The drawing under review shows one solid part. Ordinate dimensions are in mm from its lowest x, y, z. Round coordinates to 2 decimals unless told otherwise and drop trailing zeros. Write each loop counter-clockwise with the first axis right and the second up, starting at its lowest first coordinate (ties: lowest second). Pieces come first, ordered by that corner, then holes.
Item 1: Add section A-A (y = 9). State how many separate pieces and enclosed holes the cut face has, plus the area to 3 significant figures.
Item 2: Add section D-D (z = 6.55). Give the boundary of the cut face in (x, y), plus the area to 3 significant figures.
Item 3: Add section C-C (y = 5.75). Give the boundary of the cut face in (x, z).
Item 4: Clearance check with flat-ended pins moving along their axes: pin 1 Ø1 at (x, y) = (25, 7.5) entering from -Z; pin 2 Ø2 at (x, y) = (10, 3) entering from -Z; pin 3 Ø0.8 at (x, z) = (5, 38.5) entering from +Y; pin 4 Ø0.6 at (x, z) = (20, 43) entering from +Y. State where each tip first meets the part, or that it passes through.
Item 5: Draft analysis for pull direction Z (two halves, no side actions). For the marked faces 1, 2, 3 and 4, state which applies: +Z half, -Z half, draft (parallel to the pull), parting line (faces both ways), or undercut.
Item 6: To check wall thickness, follow L1, parallel to X at y = 3.25, z = 6.55; L2, parallel to Z at x = 34, y = 1.75; L3, parallel to X at y = 0.8, z = 37.55. State the ranges of each line that lie inside material, in increasing order.
Item 7: Add section B-B (x = 4.05). Give the boundary of the cut face in (y, z).
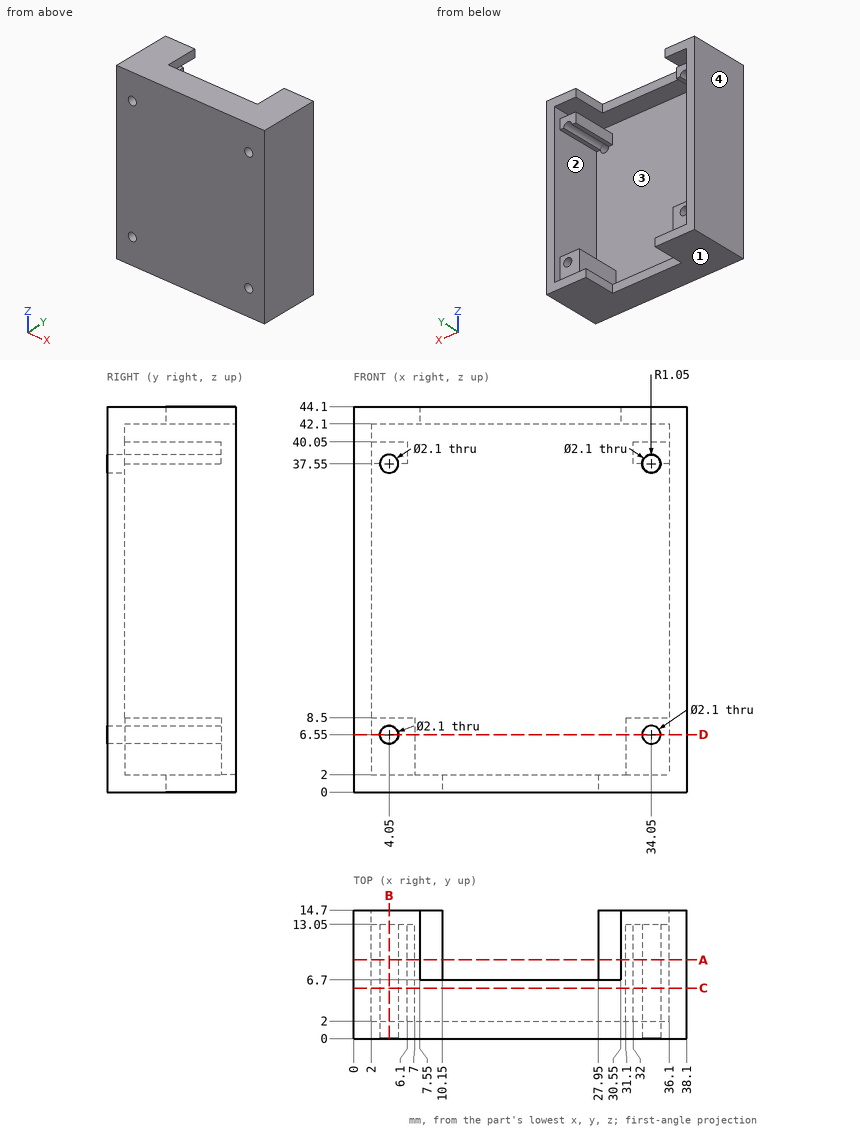
Numbers:
1. separate pieces: 2
1. enclosed holes: 2
1. area: 306 mm2
2. outline: (0, 0) - (3, 0) - (3, 13.05) - (2, 13.05) - (2, 14.7) - (0, 14.7) - close; (5.1, 0) - (33, 0) - (33, 13.05) - (31.1, 13.05) - (31.1, 2) - (7, 2) - (7, 13.05) - (5.1, 13.05) - close; (35.1, 0) - (38.1, 0) - (38.1, 14.7) - (36.1, 14.7) - (36.1, 13.05) - (35.1, 13.05) - close
2. area: 183 mm2
3. outline: (0, 0) - (38.1, 0) - (38.1, 44.1) - (0, 44.1) - close; hole (2, 8.5) - (7, 8.5) - (7, 2) - (31.1, 2) - (31.1, 8.5) - (36.1, 8.5) - (36.1, 37.55) - (35.1, 37.55) arc R1.05 ccw to (33, 37.55) - (32, 37.55) - (32, 40.05) - (36.1, 40.05) - (36.1, 42.1) - (2, 42.1) - (2, 40.05) - (6.1, 40.05) - (6.1, 37.55) - (5.1, 37.55) arc R1.05 ccw to (3, 37.55) - (2, 37.55) - close; hole circle Ø2.1 at (4.05, 6.55); hole circle Ø2.1 at (34.05, 6.55)
4. pin 1: passes through
4. pin 2: stops at z = 0
4. pin 3: stops at y = 13.05
4. pin 4: stops at y = 6.7
5. face 1: -Z half
5. face 2: undercut
5. face 3: undercut
5. face 4: draft
6. L1: x = 0 to 3, 5.1 to 7, 31.1 to 33, 35.1 to 38.1
6. L2: z = 0 to 5.5, 7.6 to 36.5, 38.6 to 44.1
6. L3: x = 0 to 3, 5.1 to 33, 35.1 to 38.1
7. outline: (0, 0) - (14.7, 0) - (14.7, 2) - (13.05, 2) - (13.05, 5.5) - (0, 5.5) - close; (0, 7.6) - (13.05, 7.6) - (13.05, 8.5) - (2, 8.5) - (2, 36.5) - (0, 36.5) - close; (0, 38.6) - (13.05, 38.6) - (13.05, 40.05) - (2, 40.05) - (2, 42.1) - (14.7, 42.1) - (14.7, 44.1) - (0, 44.1) - close
